Geometry: final body of the model. Coordinates: model frame, mm. Face numbers are marked on the shaded views. A direction names the side the tool comes from. Give positions to 0.01 mm unless a question says otherwise; leave off trailing zeros. Loops run counter-clockwise (first coordinate to the right, second up) from the corner with the lowest first, then second, coordinate; pieces in that order, holes last. Notation, with made-up numbers: (87, 30.25) - (113, 30.25) arc R36 ccw to (113, 68.25) - close; hole circle Ø9 at (-24, -27.5). An arc over 180 degrees is marked (long way). Use CSV: the item, a comma, the result in double quotes. Start each with the question number.
```python
from build123d import *

# Parameters (mm, degrees)
BOSS_EXTRUDE1_DEPTH = 15
SKETCH4_R           = 8.000000000000002
SKETCH4_R_2         = 7.999999999999998
BOSS_EXTRUDE2_DEPTH = 15
SKETCH5_R           = 5.000000000000004
SKETCH5_R_2         = 5.0000000000000036
CUT_EXTRUDE2_DEPTH  = 15
FILLET2_R           = 15
FILLET3_R           = 2
FILLET4_R           = 2
BOSS_EXTRUDE3_DEPTH = 3
CUT_EXTRUDE3_REACH  = 76.188
SKETCH10_R          = 1.5000000000000007
SKETCH10_R_2        = 1.500000000000004
BOSS_EXTRUDE4_DEPTH = 10.000000000000002
BOSS_EXTRUDE5_DEPTH = 3
CUT_EXTRUDE5_REACH  = 90.637
FILLET5_R           = 1
FILLET6_R           = 2
CUT_EXTRUDE6_REACH  = 80.013
FILLET7_R           = 6
FILLET8_R           = 6
FILLET9_R           = 2
CUT_EXTRUDE7_DEPTH  = 15
FILLET10_R          = 2


# Some blends are built 0.0001 mm under size
with BuildPart() as part:
    # Sketch1 → Boss-Extrude1 (new body)
    with BuildSketch(Plane.XY):
        Polygon((-17.948335406616224, 38.357764788911155), (-17.948335406616224, -1.642235211088847), (-9.948335406616222, -1.6422352110888458), (-9.948335406616222, 38.35776478891115), align=None)
        Polygon((52.051664593383784, -1.6422352110888379), (52.051664593383784, -9.642235211088838), (-17.948335406616224, -9.642235211088838), (-17.948335406616224, -1.642235211088847), align=None)
        Polygon((44.051664593383784, 38.35776478891116), (44.051664593383784, -1.6422352110888392), (52.05166459338378, -1.6422352110888379), (52.051664593383784, 38.35776478891116), align=None)
    extrude(amount=BOSS_EXTRUDE1_DEPTH)

    # Sketch4 → Boss-Extrude2 (add)
    with BuildSketch(Plane.XY.offset(15)):
        with Locations((-12.948335406616222, -9.642235211088838)):
            Circle(SKETCH4_R)
        with Locations((47.05166459338378, -9.64223521108884)):
            Circle(SKETCH4_R_2)
    extrude(amount=-BOSS_EXTRUDE2_DEPTH)

    # Sketch5 → Cut-Extrude2 (cut)
    with BuildSketch(Plane.XY.offset(15)):
        with Locations((-12.948335406616222, -9.642235211088838)):
            Circle(SKETCH5_R)
        with Locations((47.05166459338378, -9.642235211088837)):
            Circle(SKETCH5_R_2)
    extrude(amount=-CUT_EXTRUDE2_DEPTH, mode=Mode.SUBTRACT)

    # Fillet2
    fillet2_edges = [part.edges().sort_by_distance(p)[0] for p in [
        (-17.948335406616224, -3.397237212690439, 7.5),
        (52.051664593383784, -3.3972372126904498, 7.5),
    ]]
    fillet(fillet2_edges, radius=FILLET2_R)

    # Fillet3
    fillet3_edges = [part.edges().sort_by_distance(p)[0] for p in [
        (-4.94833540661622, -9.642235211088838, 7.5),
        (39.05166459338378, -9.642235211088838, 7.5),
    ]]
    fillet(fillet3_edges, radius=FILLET3_R)

    # Fillet4
    fillet4_edges = [part.edges().sort_by_distance(p)[0] for p in [
        (-9.948335406616222, -1.6422352110888463, 7.5),
        (44.051664593383784, -1.6422352110888392, 7.5),
    ]]
    fillet(fillet4_edges, radius=FILLET4_R)

    # Sketch6 → Boss-Extrude3 (add)
    with BuildSketch(Plane(origin=(3.327e-14, 38.35776478891114, 0), x_dir=(1, -4.3e-16, 0), z_dir=(4.3e-16, 1, 0))):
        Polygon((-22.948335406616234, 0), (57.05166459338378, 0), (57.05166459338378, -20), (-22.948335406616227, -20), align=None)
    extrude(amount=BOSS_EXTRUDE3_DEPTH)

    # Sketch10 → Cut-Extrude3 (cut, up to next)
    with BuildSketch(Plane(origin=(2.1e-16, -1.6422352110888447, 0), x_dir=(1, 1.3e-16, 0), z_dir=(-1.3e-16, 1, 0)), mode=Mode.PRIVATE) as cut_extrude3_sk1:
        with Locations(Location((2.0516645933837814, -6, 0), (0, 0, 180))):
            Circle(SKETCH10_R)
    cut_extrude3_tool1 = extrude(cut_extrude3_sk1.sketch, amount=-CUT_EXTRUDE3_REACH, mode=Mode.PRIVATE) & part.part
    # Sketch10 → Cut-Extrude3 (cut, up to next)
    with BuildSketch(Plane(origin=(2.1e-16, -1.6422352110888447, 0), x_dir=(1, 1.3e-16, 0), z_dir=(-1.3e-16, 1, 0)), mode=Mode.PRIVATE) as cut_extrude3_sk2:
        with Locations(Location((17.05166459338378, -3, 0), (0, 0, 180))):
            Circle(SKETCH10_R)
    cut_extrude3_tool2 = extrude(cut_extrude3_sk2.sketch, amount=-CUT_EXTRUDE3_REACH, mode=Mode.PRIVATE) & part.part
    # Sketch10 → Cut-Extrude3 (cut, up to next)
    with BuildSketch(Plane(origin=(2.1e-16, -1.6422352110888447, 0), x_dir=(1, 1.3e-16, 0), z_dir=(-1.3e-16, 1, 0)), mode=Mode.PRIVATE) as cut_extrude3_sk3:
        with Locations(Location((32.051664593383784, -6, 0), (0, 0, 180))):
            Circle(SKETCH10_R_2)
    cut_extrude3_tool3 = extrude(cut_extrude3_sk3.sketch, amount=-CUT_EXTRUDE3_REACH, mode=Mode.PRIVATE) & part.part
    add(cut_extrude3_tool1.solids().sort_by_distance((2.051665, -1.642235, 6))[0], mode=Mode.SUBTRACT)
    add(cut_extrude3_tool2.solids().sort_by_distance((17.051665, -1.642235, 3))[0], mode=Mode.SUBTRACT)
    add(cut_extrude3_tool3.solids().sort_by_distance((32.051665, -1.642235, 6))[0], mode=Mode.SUBTRACT)

    # Sketch11 → Boss-Extrude4 (add)
    with BuildSketch(Plane.XZ.offset(-38.35776478891114)):
        Polygon((24.55166459338377, 7.3e-16), (9.551664593383764, -2.02e-15), (9.551664593383764, 8.311370234309834), (24.551664593383766, 8.311370234309837), align=None)
    extrude(amount=BOSS_EXTRUDE4_DEPTH)

    # Sketch12 → Boss-Extrude5 (add)
    with BuildSketch(Plane(origin=(1.794e-14, 41.35776478891114, 0), x_dir=(1, -4.3e-16, 0), z_dir=(4.3e-16, 1, 0))):
        Polygon((-22.948335406616234, 0), (-28.94833540661623, -3), (-28.94833540661623, -17), (-22.948335406616227, -20), align=None)
        Polygon((57.05166459338377, -20.000000000000057), (63.05166459338377, -16.999999999999943), (63.05166459338377, -2.9999999999999574), (57.05166459338377, 0), align=None)
    extrude(amount=-BOSS_EXTRUDE5_DEPTH)

    # Sketch13 → Cut-Extrude5 (cut, up to next)
    with BuildSketch(Plane(origin=(1.794e-14, 41.35776478891114, 0), x_dir=(1, -4.3e-16, 0), z_dir=(4.3e-16, 1, 0)), mode=Mode.PRIVATE) as cut_extrude5_sk1:
        Polygon((59.05166459338377, -6), (61.05166459338377, -6), (61.05166459338378, -14), (59.05166459338377, -14), align=None)
    cut_extrude5_tool1 = extrude(cut_extrude5_sk1.sketch, amount=-CUT_EXTRUDE5_REACH, mode=Mode.PRIVATE) & part.part
    # Sketch13 → Cut-Extrude5 (cut, up to next)
    with BuildSketch(Plane(origin=(1.794e-14, 41.35776478891114, 0), x_dir=(1, -4.3e-16, 0), z_dir=(4.3e-16, 1, 0)), mode=Mode.PRIVATE) as cut_extrude5_sk2:
        Polygon((-26.948335406616234, -5.999999999999999), (-24.94833540661623, -6), (-24.94833540661623, -14.000000000000002), (-26.948335406616234, -14.000000000000002), align=None)
    cut_extrude5_tool2 = extrude(cut_extrude5_sk2.sketch, amount=-CUT_EXTRUDE5_REACH, mode=Mode.PRIVATE) & part.part
    add(cut_extrude5_tool1.solids().sort_by_distance((60.051665, 41.357765, 10))[0], mode=Mode.SUBTRACT)
    add(cut_extrude5_tool2.solids().sort_by_distance((-25.948335, 41.357765, 10))[0], mode=Mode.SUBTRACT)

    # Fillet5
    fillet5_edges = [part.edges().sort_by_distance(p)[0] for p in [
        (59.05166459338379, 39.85776478891111, 6),
        (61.05166459338379, 39.85776478891111, 6),
        (61.0516645933838, 39.85776478891111, 14),
        (59.05166459338379, 39.85776478891111, 14),
        (-26.948335406616216, 39.857764788911155, 14.000000000000002),
        (-24.948335406616213, 39.857764788911155, 14.000000000000002),
        (-24.948335406616213, 39.857764788911155, 6),
        (-26.948335406616216, 39.857764788911155, 5.999999999999999),
    ]]
    fillet(fillet5_edges, radius=FILLET5_R - 0.0001)  # a hair under: the kernel refuses the full size

    # Fillet6
    fillet6_edges = [part.edges().sort_by_distance(p)[0] for p in [
        (-22.948335406616202, 39.85776478891115, 0),
        (-22.948335406616195, 39.85776478891115, 20),
        (57.05166459338381, 39.85776478891112, 20),
        (57.05166459338381, 39.85776478891112, 0),
        (-28.948335406616213, 39.857764788911155, 17),
        (-28.948335406616213, 39.857764788911155, 3),
        (63.05166459338379, 39.85776478891111, 2.9999999999999574),
        (63.05166459338379, 39.85776478891111, 16.999999999999943),
    ]]
    fillet(fillet6_edges, radius=FILLET6_R)

    # Sketch14 → Cut-Extrude6 (cut, up to next)
    with BuildSketch(Plane(origin=(0, 0, 0), x_dir=(-1, 0, 0), z_dir=(0, 0, -1)), mode=Mode.PRIVATE) as cut_extrude6_sk1:
        Polygon((-42.051664593383784, -18.97236223001103), (-52.05166459338378, -18.97236223001103), (-49.55166459338378, -13.972362230011036), (-44.55166459338378, -13.972362230011036), align=None)
    cut_extrude6_tool1 = extrude(cut_extrude6_sk1.sketch, amount=-CUT_EXTRUDE6_REACH, mode=Mode.PRIVATE) & part.part
    # Sketch14 → Cut-Extrude6 (cut, up to next)
    with BuildSketch(Plane(origin=(0, 0, 0), x_dir=(-1, 0, 0), z_dir=(0, 0, -1)), mode=Mode.PRIVATE) as cut_extrude6_sk2:
        Polygon((17.948335406616224, -18.972362230011036), (7.948335406616221, -18.972362230011036), (10.448335406616224, -13.972362230011036), (15.448335406616224, -13.972362230011036), align=None)
    cut_extrude6_tool2 = extrude(cut_extrude6_sk2.sketch, amount=-CUT_EXTRUDE6_REACH, mode=Mode.PRIVATE) & part.part
    add(cut_extrude6_tool1.solids().sort_by_distance((47.051665, -16.75014, 0))[0], mode=Mode.SUBTRACT)
    add(cut_extrude6_tool2.solids().sort_by_distance((-12.948335, -16.75014, 0))[0], mode=Mode.SUBTRACT)

    # Fillet7
    fillet7_edges = [part.edges().sort_by_distance(p)[0] for p in [
        (24.55166459338378, 28.35776478891113, 4.155685117154919),
        (9.551664593383776, 28.357764788911137, 4.155685117154916),
    ]]
    fillet(fillet7_edges, radius=FILLET7_R)

    # Fillet8
    # the kernel refuses this fillet: 6 mm, written as the material it adds along each edge
    with BuildSketch(Plane(origin=(24.551664593383784, 38.35776478891113, 8.311370234309837), x_dir=(1, -1.22e-15, 4.3e-16), z_dir=(4.3e-16, 0, -1))) as fillet8_piece_1:
        with BuildLine():
            CenterArc((5.832159566204599, 6), FILLET8_R, 189.5940682268561, 80.40593177314383)
            Line((-0.08392021689509223, 5.000000000000448), (-0.675528195205062, 4.90000000000049))
            ThreePointArc((-0.675528195205062, 4.90000000000049), (-0.5999999999999965, 4.000000000000001), (-0.6000000000000014, 7.3e-16))
            Line((-0.6000000000000014, 7.3e-16), (-7.3e-16, -0.6000000000000014))
            Line((-7.3e-16, -0.6000000000000014), (5.832159566204594, -0.6000000000000014))
            Line((5.832159566204594, -0.6000000000000014), (5.832159566204595, 0))
        make_face()
    extrude(amount=8.311370234309837)
    with BuildSketch(Plane(origin=(9.55166459338378, 38.35776478891113, -2.02e-15), x_dir=(0.01678167981240219, -0.9998591776958763, 0), z_dir=(0, 0, 1))) as fillet8_piece_2:
        with BuildLine():
            CenterArc((5.901281631719588, -5.932028346925651), FILLET8_R, 98.63250366346277, 80.40593177319276)
            Line((-0.09787343445575636, -5.831338268056363), (-0.6977889410732921, -5.8212692601694345))
            Line((-0.6977889410732921, -5.8212692601694345), (-0.5999155066175272, 0.01006900788744134))
            Line((-0.5999155066175272, 0.01006900788744134), (0.01006900788744131, 0.5999155066175255))
            ThreePointArc((0.01006900788744131, 0.5999155066175255), (4.009505718670954, 0.5327887873679148), (4.9106464685856706, 0.5932028346925657))
            Line((4.9106464685856706, 0.5932028346925657), (5.000704210688756, 1e-17))
        make_face()
    extrude(amount=8.311370234309836)

    # Fillet9
    fillet9_edges = [part.edges().sort_by_distance(p)[0] for p in [
        (17.05166459338424, 38.35776478891257, 8.31137023431),
    ]]
    fillet(fillet9_edges, radius=FILLET9_R)

    # Sketch15 → Cut-Extrude7 (cut)
    with BuildSketch(Plane(origin=(0, 0, 0), x_dir=(-1, 0, 0), z_dir=(0, 0, -1))):
        Polygon((-12.43286243986677, 34.35776478891113), (-14.742263516625279, 38.35776478891114), (-19.36106567014228, 38.35776478891114), (-21.67046674690079, 34.35776478891113), (-19.36106567014228, 30.357764788911126), (-14.742263516625275, 30.357764788911126), align=None)
    extrude(amount=-CUT_EXTRUDE7_DEPTH, mode=Mode.SUBTRACT)

    # Fillet10
    fillet10_edges = [part.edges().sort_by_distance(p)[0] for p in [
        (-17.948335406616224, 38.357764788911155, 7.5),
        (-9.948335406616222, 38.35776478891115, 7.5),
        (44.051664593383784, 38.35776478891116, 7.5),
        (52.051664593383784, 38.35776478891116, 7.5),
        (48.051664593383784, 38.35776478891116, 15),
        (-13.948335406616224, 38.357764788911155, 15),
    ]]
    fillet(fillet10_edges, radius=FILLET10_R)


solid = part.part
```
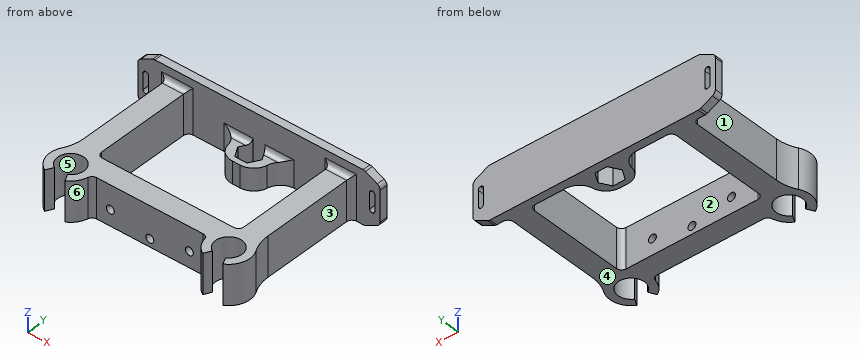
Item 1: Ray query, probe 1 along Y at (x, z) = (16, 1.75); probe 2 along Y at (x, z) = (0, 12.5); probe 3 along X at (y, z) = (31, 12.25). Return the intervals inside material, ascending.
Item 2: Section B-B (z = 12). Give the number of separate pieces and of enclosed holes in the cut face, plus the area to 3 significant figures.
Item 3: Section A-A (x = 35). Output: boundary loops of the cut face in (y, z).
Item 4: Reachability of the marked faces 1, 2 and 3 from +Z, -Z, +X, -X, +Y, -Y: full face, straight path, thin tool, end or side. Return the list, or none.
Item 5: Pin query (flat end, axial travel): pin 1 Ø4 at (x, z) = (2.05, 6) entering from -Y; pin 2 Ø11.5 at (x, y) = (47.05, -9.64) entering from +Z; pin 3 Ø2 at (y, z) = (19, 5) entering from -X. Return the tip coordinate at first contact, or that it passes through.
Item 6: Mould query, pull axis Y, two halves, no side actions, for the marked faces 4, 5 and 6. Classes: pulls with the +Y half, pulls with the -Y half, needs draft (parallel to the pull), parting line crosses it, or undercut.
Outcome:
1,probe 1,"y = -9.64 to -1.64, 28.36 to 30.36, 38.36 to 41.36"
1,probe 2,"y = -9.64 to -1.64, 38.36 to 41.36"
1,probe 3,"x = -17.95 to -9.95, 44.05 to 52.05"
2,separate pieces,"3"
2,enclosed holes,"1"
2,area,"1,510 mm2"
3,outline,"(-9.64, 0) - (-1.64, 0) - (-1.64, 15) - (-9.64, 15) - close; (38.36, 0) - (41.36, 0) - (41.36, 20) - (38.36, 20) - close"
4,face 1,"+Z, -Z, -X"
4,face 2,"+Z, -Z"
4,face 3,"+Z, -Z, +X"
5,pin 1,"stops at y = -9.64"
5,pin 2,"stops at z = 15"
5,pin 3,"stops at x = -17.95"
6,face 4,"needs draft"
6,face 5,"undercut"
6,face 6,"pulls with the -Y half"
